from build123d import *

# Parameters (mm, degrees)
BOSS_EXTRUDE1_DEPTH                        = 3
FILLET1_R                                  = 1
SKETCH2_R                                  = 1.6
MOTOR_DRIVER_HOLES_DEPTH                   = 183.893494651
SKETCH3_W                                  = 20
SKETCH3_H                                  = 15
MOTOR_DRIVER_ROUTING_POCKET_DEPTH          = 183.893494651
MOTOR_DRIVER_ROUTING_POCKET_FILLETS_R      = 1
MOTOR_DRIVER_ROUTING_POCKET_FILLETS_OF_M_R = 1
SKETCH5_W                                  = 35
SKETCH5_H                                  = 76
BATTERY_SEAT_DEPTH                         = 183.893494651
SKETCH6_R                                  = 1.6
MICROCONTROLLER_STANDOFF_HOLES_DEPTH       = 183.893494651
SKETCH8_R                                  = 1.6
PLATE_STANDOFF_HOLES_DEPTH                 = 183.893494651


with BuildPart() as part:
    # Sketch1 → Boss-Extrude1 (new body)
    with BuildSketch(Plane(origin=(0, 0, 0), x_dir=(1, 0, 0), z_dir=(0, 1, 0))):
        Polygon((0, 52), (0, -52), (87.617056359, -52), (106.15, -84.1), (143.85, -84.1), (162.382943641, -52), (162.382943641, 52), (143.85, 84.1), (106.15, 84.1), (87.617056359, 52), align=None)
    extrude(amount=BOSS_EXTRUDE1_DEPTH)

    # Fillet1
    fillet1_edges = [part.edges().sort_by_distance(p)[0] for p in [
        (0, 1.5, 52),
        (0, 1.5, -52),
    ]]
    fillet(fillet1_edges, radius=FILLET1_R)

    # Sketch2 → Motor Driver Holes (cut, through all)
    with BuildSketch(Plane(origin=(0, 3, 0), x_dir=(1, 0, 0), z_dir=(0, 1, 0))):
        with Locations(Location((4, 18.5, 0), (0, 0, 270))):
            Circle(SKETCH2_R)
        with Locations(Location((41, 18.5, 0), (0, 0, 270))):
            Circle(SKETCH2_R)
        with Locations(Location((4, -18.5, 0), (0, 0, 270))):
            Circle(SKETCH2_R)
        with Locations(Location((41, -18.5, 0), (0, 0, 270))):
            Circle(SKETCH2_R)
    extrude(amount=-MOTOR_DRIVER_HOLES_DEPTH, mode=Mode.SUBTRACT)

    # Sketch3 → Motor Driver Routing Pocket (cut, through all)
    with BuildSketch(Plane(origin=(0, 3, 0), x_dir=(1, 0, 0), z_dir=(0, 1, 0))):
        with Locations((28, 32.5)):
            Rectangle(SKETCH3_W, SKETCH3_H)
    motor_driver_routing_pocket = extrude(amount=-MOTOR_DRIVER_ROUTING_POCKET_DEPTH, mode=Mode.SUBTRACT)

    # Motor Driver Routing Pocket Fillets
    motor_driver_routing_pocket_fillets_edges = [part.edges().sort_by_distance(p)[0] for p in [
        (38, 1.5, -40),
        (38, 1.5, -25),
        (18, 1.5, -25),
        (18, 1.5, -40),
    ]]
    fillet(motor_driver_routing_pocket_fillets_edges, radius=MOTOR_DRIVER_ROUTING_POCKET_FILLETS_R)

    # Mirror1: Motor Driver Routing Pocket across plane
    add(motor_driver_routing_pocket.mirror(Plane.XY), mode=Mode.SUBTRACT)

    # Motor Driver Routing Pocket Fillets of M
    motor_driver_routing_pocket_fillets_of_m_edges = [part.edges().sort_by_distance(p)[0] for p in [
        (38, 1.5, 40),
        (38, 1.5, 25),
        (18, 1.5, 25),
        (18, 1.5, 40),
    ]]
    fillet(motor_driver_routing_pocket_fillets_of_m_edges, radius=MOTOR_DRIVER_ROUTING_POCKET_FILLETS_OF_M_R)

    # Sketch5 → Battery Seat (cut, through all)
    with BuildSketch(Plane(origin=(0, 3, 0), x_dir=(1, 0, 0), z_dir=(0, 1, 0))):
        with Locations((67.5, 0)):
            Rectangle(SKETCH5_W, SKETCH5_H)
    extrude(amount=-BATTERY_SEAT_DEPTH, mode=Mode.SUBTRACT)

    # Sketch6 → Microcontroller Standoff Holes (cut, through all)
    with BuildSketch(Plane(origin=(0, 3, 0), x_dir=(1, 0, 0), z_dir=(0, 1, 0))):
        with Locations(Location((136, -38.75, 0), (0, 0, 270))):
            Circle(SKETCH6_R)
        with Locations(Location((151.24, 12.05, 0), (0, 0, 270))):
            Circle(SKETCH6_R)
        with Locations(Location((102.98, 13.32, 0), (0, 0, 270))):
            Circle(SKETCH6_R)
    extrude(amount=-MICROCONTROLLER_STANDOFF_HOLES_DEPTH, mode=Mode.SUBTRACT)

    # Sketch8 → Plate Standoff Holes (cut, through all)
    with BuildSketch(Plane(origin=(0, 3, 0), x_dir=(1, 0, 0), z_dir=(0, 1, 0))):
        with Locations(Location((5, 27, 0), (0, 0, 270))):
            Circle(SKETCH8_R)
        with Locations(Location((5, -27, 0), (0, 0, 270))):
            Circle(SKETCH8_R)
        with Locations(Location((98, -55, 0), (0, 0, 270))):
            Circle(SKETCH8_R)
        with Locations(Location((98, 55, 0), (0, 0, 270))):
            Circle(SKETCH8_R)
        with Locations(Location((152, -55, 0), (0, 0, 270))):
            Circle(SKETCH8_R)
        with Locations(Location((152, 55, 0), (0, 0, 270))):
            Circle(SKETCH8_R)
    extrude(amount=-PLATE_STANDOFF_HOLES_DEPTH, mode=Mode.SUBTRACT)


solid = part.part
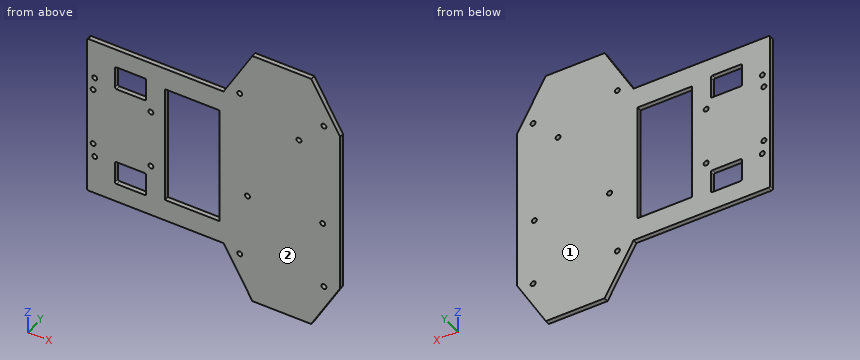
For this review, take the finished solid that the model builds, in its own axes (mm). Face numbers are marked on the shaded views. Round coordinates to 2 decimals unless told otherwise and drop trailing zeros. Order: outer loops, then holes, each group sorted by start corner. A loop starts at its lowest first (then second) coordinate and runs counter-clockwise, first axis right, second up. Notation, with made-up numbers: (50.5, 56) -> (57.5, 56) arc R21 cw to (57.5, 83) -> close; hole circle Ø2 at (51.25, -18). An arc over 180 degrees is marked (long way). Write item = value, one per line. Start each with the question number.
1) Take a section at C-C on y = 1.8. Count the separate pieces of the cut face and the enclosed holes in it, plus the area to 3 significant figures.
2) Take a section at A-A on z = 35. State the section outline as (x, y) points, plus the area to 3 significant figures.
3) To check wall thickness, follow line 1 (X direction, y = 0.6, z = 18.5); line 2 (Z direction, x = 28, y = 2.45); line 3 (X direction, y = 1.8, z = 29.5). State the ranges of each line that lie inside material, in increasing order. Write a range as from..to.
4) Insertion check: pin 1 (4 mm diameter, centred on x = 41, z = -18.5, fed in from -Y); pin 2 (1.5 mm diameter, centred on x = 28.5, y = 2, fed in from +Z); pin 3 (1.9 mm diameter, centred on x = 98, z = 55, fed in from +Y). Each pin has a flat end and moves straight along its axis. Give the tip position at first contact, or say it passes through.
5) Take a section at B-B on x = 25. State the section outline as (y, z) points, plus the area to 3 significant figures.
6) The part is to be moulded in two halves that separate along Y. For the marked faces 1 and 2, say which applies: +Y half, -Y half, draft (parallel to the pull), parting line (faces both ways), or undercut.
7) Take a section at D-D on z = -60. State the section outline as (x, y) points, plus the area to 3 significant figures.
Verdict:
q1.separate_pieces = 1
q1.enclosed_holes = 16
q1.area = 17,100 mm2
q2.outline = (0, 0) -> (18, 0) -> (18, 3) -> (0, 3) -> close; (38, 0) -> (50, 0) -> (50, 3) -> (38, 3) -> close; (85, 0) -> (162.38, 0) -> (162.38, 3) -> (85, 3) -> close
q2.area = 322 mm2
q3.line_1 = 0..2.4, 5.6..39.4, 42.6..50, 85..162.38
q3.line_2 = -52..-40, -25..25, 40..52
q3.line_3 = 0..18, 38..50, 85..162.38
q4.pin_1 = 0
q4.pin_2 = 52
q4.pin_3 = through
q5.outline = (0, -52) -> (3, -52) -> (3, -40) -> (0, -40) -> close; (0, -25) -> (3, -25) -> (3, 25) -> (0, 25) -> close; (0, 40) -> (3, 40) -> (3, 52) -> (0, 52) -> close
q5.area = 222 mm2
q6.face_1 = +Y half
q6.face_2 = -Y half
q7.outline = (92.24, 0) -> (157.76, 0) -> (157.76, 3) -> (92.24, 3) -> close
q7.area = 197 mm2
